Here's how the part is built. I have some questions about the finished solid (model axes, mm). Face numbers are marked on the shaded views. Give positions to 0.01 mm unless a question says otherwise; leave off trailing zeros. Order: outer loops, then holes, each group sorted by start corner. A loop starts at its lowest first (then second) coordinate and runs counter-clockwise, first axis right, second up.
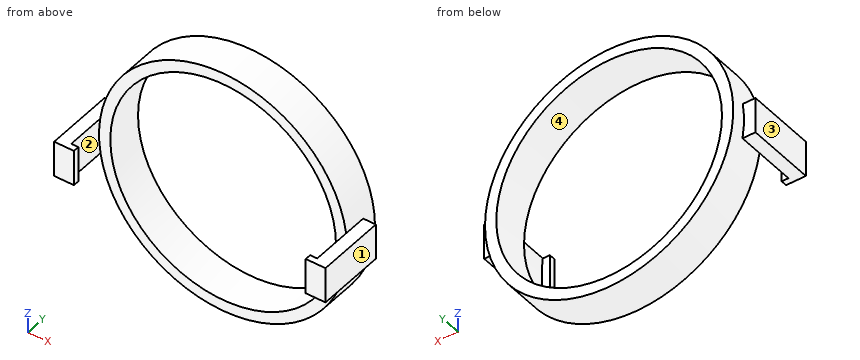
Autodesk Inventor part; units mm, degrees
ref_plane "YZ Plane" through (0, 0, 0) normal (1, 0, 0) x (0, 1, 0)
ref_plane "XZ Plane" through (0, 0, 0) normal (0, 1, 0) x (-1, 0, 0)
ref_plane "XY Plane" through (0, 0, 0) normal (0, 0, 1) x (1, 0, 0)
ref_plane "Work Plane11" through (0, 7, 0) normal (0, 1, 0) x (1, 0, 0)
sketch "Sketch16" plane through (0, 7, 0) normal (0, 1, 0) x (1, 0, 0)
  circle A0 centre (0, 0) radius 22
  circle A1 centre (0, 0) radius 20
  circle A2 centre (0, 0) radius 18.4
  dimension "d44" = 36.8
extrude "Extrusion13" add sketch "Sketch16" along normal blind 6.7 contours A0
ref_plane "Work Plane3" through (24.0456, 0, 22.026) normal (1, 0, 0) x (0, 0, -1)
sketch "Sketch19" plane through (24.0456, 0, 22.026) normal (1, 0, 0) x (0, 0, -1)
  line L0 (19.05, 11.1125) -> (25.4, 11.1125)
  line L1 (25.4, 11.1125) -> (25.4, 7.9375)
  line L2 (25.4, 7.9375) -> (19.05, 7.9375)
  line L3 (19.05, 7.9375) -> (19.05, 11.1125)
  point P0 (22.026, 0)
extrude "Extrusion15" add sketch "Sketch19" against normal blind 3
sketch "Sketch20" plane through (24.0456, 7.9375, -3.374) normal (0, -1, 0) x (1, 0, 0)
  line L0 (0, 6.35) -> (0, 0)
  line L1 (0, 6.35) -> (0, 0)
  line L2 (0, 0) -> (-2.3058, 0)
  line L3 (0, 0) -> (-2.3058, 0)
  arc A0 (-38.8494, -12.9001) -> (-38.8494, 19.6481) centre (-24.0456, 3.374) ccw
  arc A1 (-2.3058, 0) -> (-2.3058, 6.7481) centre (-24.0456, 3.374) ccw
  line L4 (0, 6.35) -> (-2.2478, 6.35)
  line L5 (0, 6.35) -> (-2.2478, 6.35)
  point P0 (-3, 0)
  point P1 (-3, 6.35)
extrude "Extrusion16" add sketch "Sketch20" along normal blind 9
sketch "Sketch21" plane through (24.0456, 0, 22.026) normal (1, 0, 0) x (0, 0, -1)
  line L0 (25.4, 0) -> (19.05, 0)
  line L1 (19.05, 11.1125) -> (19.05, -1.0625)
  line L2 (19.05, 0) -> (19.05, -1.0625)
  line L3 (25.4, 11.1125) -> (25.4, -1.0625)
  line L4 (19.05, -1.0625) -> (25.4, -1.0625)
  line L5 (25.4, -1.0625) -> (25.4, 0)
  point P0 (22.026, 0)
ref_plane "Work Plane4" through (-24.0451, 0, 16.0514) normal (-1, 0, 0) x (0, 0, 1)
sketch "Sketch23" plane through (-24.0451, 0, 16.0514) normal (-1, 0, 0) x (0, 0, 1)
  line L0 (-19.4254, 11.1125) -> (-19.4254, 0)
  line L1 (-13.0754, 11.1125) -> (-13.0754, -1.0625)
  line L2 (-19.4254, 11.1125) -> (-13.0754, 11.1125)
  line L3 (-13.0754, 11.1125) -> (-13.0754, 7.9375)
  line L4 (-13.0754, 7.9375) -> (-19.4254, 7.9375)
  line L5 (-19.4254, 7.9375) -> (-19.4254, 11.1125)
  point P0 (-16.0514, 0)
extrude "Extrusion17" add sketch "Sketch23" against normal blind 3
sketch "Sketch24" plane through (-24.0451, 7.9375, -3.374) normal (0, -1, 0) x (1, 0, 0)
  arc A0 (2.2473, 6.35) -> (2.3053, 0) centre (24.0451, 3.374) ccw
  line L0 (2.3053, 0) -> (0, 0)
  line L1 (0, 0) -> (0, 6.35)
  line L2 (0, 0) -> (0, 6.35)
  line L3 (0, 6.35) -> (2.2473, 6.35)
  line L4 (0, 6.35) -> (2.2473, 6.35)
  arc A1 (2.2473, 6.35) -> (2.3053, 0) centre (24.0451, 3.374) ccw
  point P0 (3, 6.35)
extrude "Extrusion18" add sketch "Sketch24" along normal blind 9
sketch "Sketch25" plane through (-24.0451, 0, 16.0514) normal (-1, 0, 0) x (0, 0, 1)
  line L0 (-19.4254, 11.1125) -> (-19.4254, -1.0625)
  line L1 (-13.0754, 0) -> (5.9486, 0)
  line L2 (-19.4254, -1.0625) -> (-13.0754, -1.0625)
  line L3 (-13.0754, -1.0625) -> (-13.0754, 0)
  line L4 (-13.0754, 0) -> (-19.4254, 0)
  line L5 (-19.4254, 0) -> (-19.4254, -1.0625)
  point P0 (-16.0514, 0)
  point P1 (0.2227, 0)
extrude "Extrusion19" add sketch "Sketch25" against normal blind 3.5
sketch "Sketch26" plane through (24.0456, 0, 22.026) normal (1, 0, 0) x (0, 0, -1)
  line L0 (25.4, 11.1125) -> (25.4, 0)
  line L1 (19.05, -1.0625) -> (25.4, -1.0625)
  line L2 (25.4, 0) -> (19.05, 0)
  line L3 (19.05, 0) -> (19.05, -1.0625)
  line L4 (19.05, -1.0625) -> (25.4, -1.0625)
  line L5 (25.4, -1.0625) -> (25.4, 0)
  point P0 (22.026, 0)
extrude "Extrusion20" add sketch "Sketch26" against normal blind 3.5
properties part number "watchBodyOneTop"
Q1. I'm going to push flat-ended pins straight in: P1, Ø2, axis at y = 11.5, z = 16, coming from the +X side; P2, Ø1.8, axis at x = 23, y = 4, coming from the +Z side; P3, Ø1, axis at y = 7, z = 15, coming from the -X side; P4, Ø6, axis at x = -4, z = -15.5, coming from the +Y side. Where does each tip first touch, or does it pass through?
Filled sheet:
P1: stops at x = 16.09
P2: stops at z = 2.98
P3: stops at x = -16.55
P4: passes through
Q2. Thinking about a two-plate mould opening in X: for the marked faces 1, 2, 3 and 4, which applies, released by +X, released by -X, zero draft, split by the parting line, or undercut?
Filled sheet:
face 1: released by +X
face 2: undercut
face 3: released by -X
face 4: undercut
Q3. If we section it at A-A on x = 0: List the corners of the cut face in (y, z) for me.
Filled sheet:
outline: (7, -22) - (13.7, -22) - (13.7, -20) - (7, -20) - close; (7, 20) - (13.7, 20) - (13.7, 22) - (7, 22) - close
Q4. If we section it at B-B on z = 0: List the corners of the cut face in (x, y) for me.
Filled sheet:
outline: (-24.05, -1.06) - (-20.55, -1.06) - (-20.55, 0) - (-22, 0) - (-22, 7) - (-20, 7) - (-20, 13.7) - (-22, 13.7) - (-22, 11.11) - (-24.05, 11.11) - close; (20, 7) - (22, 7) - (22, 0) - (20.55, 0) - (20.55, -1.06) - (24.05, -1.06) - (24.05, 11.11) - (22, 11.11) - (22, 13.7) - (20, 13.7) - close
Q5. If we section it at D-D on y = 10: List the corners of the cut face in (x, z) for me.
Filled sheet:
outline: (-24.05, -3.37) - (-21.74, -3.37) arc R22 ccw to (21.74, -3.37) - (24.05, -3.37) - (24.05, 2.98) - (21.8, 2.98) arc R22 ccw to (-21.8, 2.98) - (-24.05, 2.98) - close; hole circle Ø40 at (0, 0)
Q6. I need wall thicknesses on L1, parallel to Z at x = 0, y = 8.75; L2, parallel to X at y = 10.25, z = 0. Which ranges of each line are inside material? Lowest first, please.
Filled sheet:
L1: z = -22 to -20, 20 to 22
L2: x = -24.05 to -20, 20 to 24.05
Q7. If we section it at C-C on y = 4: List the corners of the cut face in (x, z) for me.
Filled sheet:
outline: (-24.05, -3.37) - (-21.74, -3.37) arc R22 cw to (-21.8, 2.98) - (-24.05, 2.98) - close; (21.74, -3.37) - (24.05, -3.37) - (24.05, 2.98) - (21.8, 2.98) arc R22 cw to start
